Here's how the part is built. I have some questions about the finished solid (model axes, mm). Face numbers are marked on the shaded views. Round coordinates to 2 decimals unless told otherwise and drop trailing zeros. Loops run counter-clockwise (first coordinate to the right, second up) from the corner with the lowest first, then second, coordinate; pieces in that order, holes last. Notation, with made-up numbers: M -15,-7 L 0,-7 A36 ccw 0,32 Z; hole C -4.5,23.25 d10. An arc over 180 degrees is marked long. Write each question's results on one line, items separated by ' | '. Start each with the question number.
```python
from build123d import *

# Parameters (mm, degrees)
SKETCH_1_W          = 70
SKETCH_1_H          = 70
EXTRUDE_1_DEPTH     = 3.4
SKETCH_2_W          = 30
SKETCH_2_H          = 30
CUT_EXTRUDE_1_DEPTH = 2.6
SKETCH_3_R          = 2.6
CUT_EXTRUDE_2_DEPTH = 4.4
EXTRUDE_2_DEPTH     = 3
SKETCH_6_R          = 1.6
EXTRUDE_3_DEPTH     = 0.3


with BuildPart() as part:
    # 草图1 → 凸台-拉伸1 (new body)
    with BuildSketch(Plane.XY):
        with BuildLine():
            Line((-2, 17), (0, 17))
            Line((0, 17), (0, 53))
            Line((0, 53), (-2, 53))
            ThreePointArc((-2, 53), (-4.121320344, 52.121320344), (-5, 50))
            Line((-5, 50), (-5, 20))
            ThreePointArc((-5, 20), (-4.121320344, 17.878679656), (-2, 17))
        make_face()
        with Locations((35, 35)):
            Rectangle(SKETCH_1_W, SKETCH_1_H)
        with BuildLine():
            Line((70, 53), (70, 17))
            Line((70, 17), (72, 17))
            ThreePointArc((72, 17), (74.121320344, 17.878679656), (75, 20))
            Line((75, 20), (75, 50))
            ThreePointArc((75, 50), (74.121320344, 52.121320344), (72, 53))
            Line((72, 53), (70, 53))
        make_face()
    extrude(amount=EXTRUDE_1_DEPTH)

    # 草图2 → 切除-拉伸1 (cut)
    with BuildSketch(Plane.XY.offset(3.4)):
        with Locations((35, 35)):
            Rectangle(SKETCH_2_W, SKETCH_2_H)
    extrude(amount=-CUT_EXTRUDE_1_DEPTH, mode=Mode.SUBTRACT)

    # 草图3 → 切除-拉伸2 (cut, through all)
    with BuildSketch(Plane.XY.offset(3.4)):
        with Locations((8, 62)):
            Circle(SKETCH_3_R)
        with Locations((62, 62)):
            Circle(SKETCH_3_R)
        with Locations((8, 8)):
            Circle(SKETCH_3_R)
        with Locations((62, 8)):
            Circle(SKETCH_3_R)
    extrude(amount=-CUT_EXTRUDE_2_DEPTH, mode=Mode.SUBTRACT)

    # 草图4 → 凸台-拉伸2 (add)
    with BuildSketch(Plane.XY):
        with BuildLine():
            Line((20, 44), (20, 50))
            Line((20, 50), (26, 50))
            ThreePointArc((26, 50), (24.242640687, 45.757359313), (20, 44))
        make_face()
        with BuildLine():
            Line((50, 44), (50, 50))
            Line((50, 50), (44, 50))
            ThreePointArc((44, 50), (45.757359313, 45.757359313), (50, 44))
        make_face()
        with BuildLine():
            Line((50, 20), (44, 20))
            ThreePointArc((44, 20), (45.757359313, 24.242640687), (50, 26))
            Line((50, 26), (50, 20))
        make_face()
        with BuildLine():
            Line((20, 26), (20, 20))
            Line((20, 20), (26, 20))
            ThreePointArc((26, 20), (24.242640687, 24.242640687), (20, 26))
        make_face()
    extrude(amount=EXTRUDE_2_DEPTH)

    # 草图6 → 凸台-拉伸3 (add)
    with BuildSketch(Plane.XY.offset(3)):
        with Locations((22.5, 47.5)):
            Circle(SKETCH_6_R)
        with Locations((47.5, 47.5)):
            Circle(SKETCH_6_R)
        with Locations((47.5, 22.5)):
            Circle(SKETCH_6_R)
        with Locations((22.5, 22.5)):
            Circle(SKETCH_6_R)
        Polygon((20.1, 45.5), (20.7, 45.5), (20.7, 46.1), (21.3, 46.1), (21.3, 45.5), (21.9, 45.5), (21.9, 44.9), (21.3, 44.9), (21.3, 44.3), (20.7, 44.3), (20.7, 44.9), (20.1, 44.9), align=None)
    extrude(amount=EXTRUDE_3_DEPTH)


solid = part.part
```
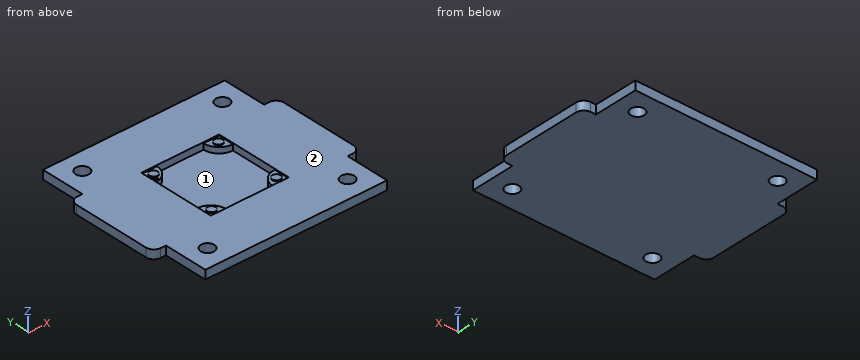
Item 1: If we section it at C-C on z = 2.05: Please give me the cut outline in (x, y), and give its area (3 significant figures).
Item 2: If we section it at D-D on y = 37: Please give me the cut outline in (x, z).
Item 3: If we mould it in two halves opening along Y, with no side actions, what happens to the marked faces 1 and 2? For each: released by +Y, released by -Y, zero draft, split by the parting line, or undercut.
Item 4: If we section it at A-A on x = 62: Please give me the cut outline in (y, z).
Item 5: I'm going to push flat-ended pins straight in: pin 1 (1 mm diameter, centred on y = 56, z = 2, fed in from +X); pin 2 (0.5 mm diameter, centred on x = 20.5, y = 45.5, fed in from +Z); pin 3 (0.6 mm diameter, centred on x = -1, z = 1.5, fed in from -Y); pin 4 (10 mm diameter, centred on x = 47.5, y = 22.5, fed in from -Z). Where does each tip first touch, or does it pass through?
Item 6: I need wall thicknesses on L1, parallel to Y at x = 62, z = 1.65; L2, parallel to Y at x = 42, z = 1.6; L3, parallel to Y at x = 20.5, z = 2.05. Which ranges of each line are inside material? Lowest first, please.
Numbers:
1) outline: M -5,20 A3 ccw -2,17 L 0,17 L 0,0 L 70,0 L 70,17 L 72,17 A3 ccw 75,20 L 75,50 A3 ccw 72,53 L 70,53 L 70,70 L 0,70 L 0,53 L -2,53 A3 ccw -5,50 Z; hole C 8,8 d5.2; hole C 8,62 d5.2; hole M 20,26 A6 cw 26,20 L 44,20 A6 cw 50,26 L 50,44 A6 cw 44,50 L 26,50 A6 cw 20,44 Z; hole C 62,8 d5.2; hole C 62,62 d5.2 | area: 4,380 mm²
2) outline: M -5,0 L 75,0 L 75,3.4 L 50,3.4 L 50,0.8 L 20,0.8 L 20,3.4 L -5,3.4 Z
3) face 1: undercut | face 2: zero draft
4) outline: M 0,0 L 5.4,0 L 5.4,3.4 L 0,3.4 Z; M 10.6,0 L 59.4,0 L 59.4,3.4 L 10.6,3.4 Z; M 64.6,0 L 70,0 L 70,3.4 L 64.6,3.4 Z
5) pin 1: x = 70 | pin 2: z = 3.3 | pin 3: y = 17 | pin 4: z = 0
6) L1: 0 to 5.4, 10.6 to 59.4, 64.6 to 70 | L2: 0 to 20, 50 to 70 | L3: 0 to 25.98, 44.02 to 70
